from build123d import *

# Parameters (mm, degrees)
F1_DEPTH = 27.5
F3_DEPTH = 20


with BuildPart() as f1:
    # F0 (on Front) → F1 (new body, symmetric)
    with BuildSketch(Plane.XZ):
        with BuildLine():
            ThreePointArc((4.057135, 8.700555), (0, -9.6), (-4.057135, 8.700555))
            ThreePointArc((-4.057135, 8.700555), (-3.113941, 11.291961), (-5.705347, 12.235155))
            ThreePointArc((-5.705347, 12.235155), (-13.179996, -2.921935), (0, -13.5))
            Line((0, -13.5), (36, -13.5))
            Line((36, -13.5), (36, -5.5))
            Line((36, -5.5), (13.5, -5.5))
            Line((13.5, -5.5), (13.5, 0))
            ThreePointArc((13.5, 0), (11.385785, 7.253545), (5.705347, 12.235155))
            ThreePointArc((5.705347, 12.235155), (3.113941, 11.291961), (4.057135, 8.700555))
        make_face()
    extrude(amount=F1_DEPTH, both=True)

    # F2 (on face) → F3 (join)
    with BuildSketch(Plane.YZ.offset(36)):
        with BuildLine():
            ThreePointArc((-26.5, 3.976179), (-27.5, -4.1), (-28.5, 3.976179))
            Line((-28.5, 3.976179), (-28.5, 10))
            Line((-28.5, 10), (-34.5, 10))
            Line((-34.5, 10), (-34.5, 0))
            ThreePointArc((-34.5, 0), (-34.241597, -1.884376), (-33.485465, -3.62963))
            Line((-33.485465, -3.62963), (-27.5, -13.5))
            Line((-27.5, -13.5), (0, -13.5))
            Line((0, -13.5), (27.5, -13.5))
            Line((27.5, -13.5), (33.485465, -3.62963))
            ThreePointArc((33.485465, -3.62963), (34.241597, -1.884376), (34.5, 0))
            Line((34.5, 0), (34.5, 10))
            Line((34.5, 10), (28.5, 10))
            Line((28.5, 10), (28.5, 3.976179))
            ThreePointArc((28.5, 3.976179), (27.5, -4.1), (26.5, 3.976179))
            Line((26.5, 3.976179), (26.5, 10))
            Line((26.5, 10), (20.5, 10))
            Line((20.5, 10), (20.5, 0))
            Line((20.5, 0), (20.5, -0.5))
            ThreePointArc((20.5, -0.5), (19.035534, -4.035534), (15.5, -5.5))
            Line((15.5, -5.5), (0, -5.5))
            Line((0, -5.5), (-15.5, -5.5))
            ThreePointArc((-15.5, -5.5), (-19.035534, -4.035534), (-20.5, -0.5))
            Line((-20.5, -0.5), (-20.5, 0))
            Line((-20.5, 0), (-20.5, 10))
            Line((-20.5, 10), (-26.5, 10))
            Line((-26.5, 10), (-26.5, 3.976179))
        make_face()
    extrude(amount=-F3_DEPTH)


solid = f1.part
Can you work these out from the model? Positions are in its coordinate system, mm. A direction names the side the tool comes from. Coordinates: 2 decimals unless noted, no trailing zeros. Write each loop counter-clockwise with the first axis right and the second up, starting at its lowest first coordinate (ties: lowest second). Pieces come first, ordered by that corner, then holes. Notation, with made-up numbers: (28, 16) - (60, 16) arc R11 cw to (60, 37) - close; hole circle Ø5 at (73.5, -9). An arc over 180 degrees is marked (long way). Return JSON: item names as keys, results as strings. Group by question number.
Item 1: We'd pull the mould along X, two halves only. Please class faces 6 (the face through (3.13, -0.39, 11.33)), 7 (the face through (26.14, 34.234, -1.91)): pulls with the +X half, pulls with the -X half, needs draft (parallel to the pull), parting line crosses it, or undercut.
Item 2: If we section it at D-D (x = 20): Write out the boundary of the cut face in (y, z).
Item 3: If we section it at C-C (z = 2.25): Write out the boundary of the cut face in (x, y).
Item 4: If we section it at A-A (z = 10.75): Write out the boundary of the cut face in (x, y), then the cut area to 3 significant figures.
Item 5: If we section it at B-B (x = 7.5): Write out the boundary of the cut face in (y, z), then the cut area to 3 significant figures.
Item 6: Please list where these lines run through material, in increasing order: probe 1 along Y at (x, z) = (25.75, 0); probe 2 along X at (y, z) = (-24.5, 9.5); probe 3 along X at (y, z) = (23, -3.5).
Item 7: Which directions (+Z, -Z, +X, -X, +Y, -Y) give clear straight access to the entire face, cutting with the end or side of a thin tool? Please do faces 1 (the face through (26, 28.5, 7)), 2 (the face through (13.5, 0, -3)), 3 (the face through (26, -20.5, 5)), 4 (the face through (26.14, -27.334, -4.097)), 5 (the face through (4, 27.5, -9)).
Item 8: I'm going to push flat-ended pins straight in: pin 1 Ø2 at (x, z) = (10, -7.5) entering from -Y; pin 2 Ø4 at (y, z) = (-26.5, 1.5) entering from +X; pin 3 Ø1.8 at (x, y) = (22, -31.5) entering from +Z. Where does each tip first touch, or does it pass through?
Return value:
{
 "1": {"face 6": "undercut", "face 7": "needs draft"},
 "2": {"outline": "(-34.5, 0) arc R7 ccw to (-33.49, -3.63) - (-27.5, -13.5) - (27.5, -13.5) - (33.49, -3.63) arc R7 ccw to (34.5, 0) - (34.5, 10) - (28.5, 10) - (28.5, 3.98) arc R4.1 cw (long way) to (26.5, 3.98) - (26.5, 10) - (20.5, 10) - (20.5, -0.5) arc R5 cw to (15.5, -5.5) - (-15.5, -5.5) arc R5 cw to (-20.5, -0.5) - (-20.5, 10) - (-26.5, 10) - (-26.5, 3.98) arc R4.1 cw (long way) to (-28.5, 3.98) - (-28.5, 10) - (-34.5, 10) - close"},
 "3": {"outline": "(-13.31, -27.5) - (-9.33, -27.5) - (-9.33, 27.5) - (-13.31, 27.5) - close; (9.33, -27.5) - (13.31, -27.5) - (13.31, 27.5) - (9.33, 27.5) - close; (16, -34.5) - (36, -34.5) - (36, -30.93) - (16, -30.93) - close; (16, -24.07) - (36, -24.07) - (36, -20.5) - (16, -20.5) - close; (16, 20.5) - (36, 20.5) - (36, 24.07) - (16, 24.07) - close; (16, 30.93) - (36, 30.93) - (36, 34.5) - (16, 34.5) - close"},
 "4": {"outline": "(-8.17, -27.5) - (-2.95, -27.5) - (-2.95, 27.5) - (-8.17, 27.5) - close; (2.95, -27.5) - (8.17, -27.5) - (8.17, 27.5) - (2.95, 27.5) - close", "area": "574 mm^2"},
 "5": {"outline": "(-27.5, -13.5) - (27.5, -13.5) - (27.5, -5.99) - (-27.5, -5.99) - close; (-27.5, 5.99) - (27.5, 5.99) - (27.5, 11.22) - (-27.5, 11.22) - close", "area": "701 mm^2"},
 "6": {"probe 1": "y = -34.5 to -31.6, -23.4 to -20.5, 20.5 to 23.4, 31.6 to 34.5", "probe 2": "x = -9.59 to -3.19, 3.19 to 9.59, 16 to 36", "probe 3": "x = -13.04 to -8.94, 8.94 to 13.5, 16 to 36"},
 "7": {"face 1": "+Z, +X, -X", "face 2": "+Z, +Y, -Y", "face 3": "+Z, +X", "face 4": "+X", "face 5": "+Z, -Z, -X, +Y"},
 "8": {"pin 1": "stops at y = -27.5", "pin 2": "stops at x = 13.5", "pin 3": "stops at z = 10"}
}
